Could you check a few things on this model? Use its own coordinates, in mm. A direction names the side the tool comes from. Round coordinates to 2 decimals unless told otherwise and drop trailing zeros. Loops run counter-clockwise (first coordinate to the right, second up) from the corner with the lowest first, then second, coordinate; pieces in that order, holes last.
from build123d import *

# Parameters (mm, degrees)
ESQUISSE1_W             = 40
ESQUISSE1_H             = 20
BOSS_EXTRU_1_DEPTH      = 10
ESQUISSE3_W             = 40
ESQUISSE3_H             = 2.1
ENL_V_MAT_EXTRU_2_DEPTH = 31
ESQUISSE4_R             = 2.05
ENL_V_MAT_EXTRU_3_DEPTH = 25.494897428
ESQUISSE5_R             = 3.1
ENL_V_MAT_EXTRU_4_DEPTH = 10


with BuildPart() as part:
    # Esquisse1 → Boss.-Extru.1 (new body)
    with BuildSketch(Plane.XY):
        Rectangle(ESQUISSE1_W, ESQUISSE1_H)
    extrude(amount=BOSS_EXTRU_1_DEPTH)

    # Esquisse3 → Enlèv. mat.-Extru.2 (cut, through all)
    with BuildSketch(Plane(origin=(0, -10, 0), x_dir=(-1, 0, 0), z_dir=(0, -1, 0))):
        with Locations((20, -5)):
            Rectangle(ESQUISSE3_W, ESQUISSE3_H)
    extrude(amount=-ENL_V_MAT_EXTRU_2_DEPTH, mode=Mode.SUBTRACT)

    # Esquisse4 → Enlèv. mat.-Extru.3 (cut, through all)
    with BuildSketch(Plane(origin=(0, 0, 0), x_dir=(-1, 0, 0), z_dir=(0, 0, -1))):
        with Locations((16, 6)):
            Circle(ESQUISSE4_R)
        with Locations((4, 6)):
            Circle(ESQUISSE4_R)
        with Locations((4, -6)):
            Circle(ESQUISSE4_R)
        with Locations((16, -6)):
            Circle(ESQUISSE4_R)
    extrude(amount=-ENL_V_MAT_EXTRU_3_DEPTH, mode=Mode.SUBTRACT)

    # Esquisse5 → Enlèv. mat.-Extru.4 (cut)
    with BuildSketch(Plane(origin=(0, 0, 0), x_dir=(-1, 0, 0), z_dir=(0, 0, -1))):
        with Locations((10, 0)):
            Circle(ESQUISSE5_R)
        with Locations(Location((-10, 0, 0), (0, 0, 180))):
            Circle(ESQUISSE5_R)
    extrude(amount=-ENL_V_MAT_EXTRU_4_DEPTH, mode=Mode.SUBTRACT)


solid = part.part
Item 1: If we section it at B-B, the plane x = -13.5: Please give me the cut outline in (y, z).
Results list:
outline: (-10, 0) - (10, 0) - (10, 3.95) - (-10, 3.95) - close; (-10, 6.05) - (10, 6.05) - (10, 10) - (-10, 10) - close
Item 2: If we section it at D-D, the plane z = 4.5: Please give me the cut outline in (x, y).
Results list:
outline: (0, -10) - (20, -10) - (20, 10) - (0, 10) - close; hole circle Ø6.2 at (10, 0)
Item 3: We'd pull the mould along Z, two halves only. Please class faces 1 (the cylindrical face through (-2.373, -7.247, 7.997)), 2 (the flat face through (-7.6, -2.4, 6.05)), 3 (the flat face through (0, 0, 10)): released by +Z, released by -Z, zero draft, split by the parting line, or undercut.
Results list:
face 1: zero draft
face 2: undercut
face 3: released by +Z
Item 4: Will this pin go through, and if not, where does the flat tip stop? pin 1 (1.1 mm diameter, centred on y = 3, z = 5, fed in from -X).
Results list:
pin 1: stops at x = 0
Item 5: If we section it at C-C, the plane x = -4: Please give me the cut outline in (y, z), then the cut area to 3 significant figures.
Results list:
outline: (-10, 0) - (-8.05, 0) - (-8.05, 3.95) - (-10, 3.95) - close; (-10, 6.05) - (-8.05, 6.05) - (-8.05, 10) - (-10, 10) - close; (-3.95, 0) - (3.95, 0) - (3.95, 3.95) - (-3.95, 3.95) - close; (-3.95, 6.05) - (3.95, 6.05) - (3.95, 10) - (-3.95, 10) - close; (8.05, 0) - (10, 0) - (10, 3.95) - (8.05, 3.95) - close; (8.05, 6.05) - (10, 6.05) - (10, 10) - (8.05, 10) - close
area: 93.2 mm2
Item 6: If I drill on line 1 along Y through (x, z) = (-4, 2.8); line 2 along Z through (x, y) = (-8.5, 6); line 3 along X through (y, z) = (0.5, 9), over which ranges is the centre line in solid material (lowest first)?
Results list:
line 1: y = -10 to -8.05, -3.95 to 3.95, 8.05 to 10
line 2: z = 0 to 3.95, 6.05 to 10
line 3: x = -20 to -13.06, -6.94 to 6.94, 13.06 to 20
Item 7: If we section it at A-A, the plane y = -6: Please give me the cut outline in (x, z), then the cut area to 3 significant figures.
Results list:
outline: (-20, 0) - (-18.05, 0) - (-18.05, 3.95) - (-20, 3.95) - close; (-20, 6.05) - (-18.05, 6.05) - (-18.05, 10) - (-20, 10) - close; (-13.95, 0) - (-6.05, 0) - (-6.05, 3.95) - (-13.95, 3.95) - close; (-13.95, 6.05) - (-6.05, 6.05) - (-6.05, 10) - (-13.95, 10) - close; (-1.95, 0) - (20, 0) - (20, 10) - (-1.95, 10) - (-1.95, 6.05) - (0, 6.05) - (0, 3.95) - (-1.95, 3.95) - close
area: 293 mm2
Item 8: For faces 4 (the flat face through (0, 0, 5)), 5 (the cylindrical face through (-13.95, -5.91, 8)), which set-ups out of +Z, -Z, +X, -X, +Y, -Y let a thin tool reach every point of the face, with its end or its side?
Results list:
face 4: -X, +Y, -Y
face 5: +Z, -Z
